Input: part model. Units: mm. Frame: model coordinates. A direction names the side the tool comes from. Give positions to 0.01 mm unless a question says otherwise; leave off trailing zeros. Order: outer loops, then holes, each group sorted by start corner. A loop starts at its lowest first (then second) coordinate and runs counter-clockwise, first axis right, second up. Notation, with made-up numbers: M -31,-5.75 L -7,-5.75 A15 ccw -7,19.25 Z; hole C 39,59 d10. An arc over 180 degrees is marked long. Use a Markdown table: item, result.
from build123d import *

# Parameters (mm, degrees)
F0_W     = 76.2
F0_H     = 76.2
F2_DEPTH = 6.35
F3_DEPTH = 6.35
F4_R     = 2.54
F6_DEPTH = 2.778125
F7_W     = 13.096875
F7_H     = 6.746875
F8_DEPTH = 0.79375


with BuildPart() as f2:
    # F0 (on Top) → F2 (new body)
    with BuildSketch(Plane.XY):
        Rectangle(F0_W, F0_H)
    extrude(amount=-F2_DEPTH)

    # F1 (on Front) → F3 (join, symmetric)
    with BuildSketch(Plane.XZ):
        with BuildLine():
            Line((18.7292598667, 44.45), (25.3953712381, 51.2535714286))
            ThreePointArc((25.3953712381, 51.2535714286), (-28.575, 28.575), (25.3953712381, 5.8964285714))
            Line((25.3953712381, 5.8964285714), (18.7292598667, 12.7))
            ThreePointArc((18.7292598667, 12.7), (-19.05, 28.575), (18.7292598667, 44.45))
        make_face()
    extrude(amount=F3_DEPTH, both=True)

    # F4
    f4_edges = [f2.edges().sort_by_distance(p)[0] for p in [
        (25.395371, 0, 51.253571),
        (18.72926, 0, 44.45),
        (18.72926, 0, 12.7),
        (25.395371, 0, 5.896429),
        (3.175, -6.35, 0),
        (3.175, 6.35, 0),
    ]]
    fillet(f4_edges, radius=F4_R)

    # F5 (on face) → F6 (join)
    with BuildSketch(Plane(origin=(0, 0, -6.35), x_dir=(1, 0, 0), z_dir=(0, 0, -1))):
        Polygon((-38.1, 14.4859375), (-38.1, 23.6140625), (-44.45, 27.2802367094), (-44.45, 10.8197632906), align=None)
        Polygon((-38.1, -23.6140625), (-38.1, -14.4859375), (-44.45, -10.8197632906), (-44.45, -27.2802367094), align=None)
    extrude(amount=-F6_DEPTH)

    # F7 (on face) → F8 (cut)
    with BuildSketch(Plane.XY):
        with Locations((-31.5515625, 9.7234375)):
            Rectangle(F7_W, F7_H)
    extrude(amount=-F8_DEPTH, mode=Mode.SUBTRACT)


solid = f2.part
1) Cut plane B-B on y = 20.5. Return loops of the section in (x, z).
Response values:
| item | result |
|---|---|
| outline | M -44.45,-6.35 L 38.1,-6.35 L 38.1,0 L -38.1,0 L -38.1,-3.57 L -44.45,-3.57 Z |
2) First-contact query: pin 1 Ø16 at (x, z) = (-8, 35.5) entering from -Y; pin 2 Ø5 at (y, z) = (18, 0.5) entering from -X; pin 3 Ø1.9 at (x, y) = (-42.5, 23) entering from +Z; pin 4 Ø7.5 at (x, y) = (-32.5, 9.5) entering from +Z. Flat tips, straight axial feed; report the tip coordinate or a pass-through.
Response values:
| item | result |
|---|---|
| pin 1 | passes through |
| pin 2 | stops at x = -38.1 |
| pin 3 | stops at z = -3.57 |
| pin 4 | stops at z = 0 |
3) Cut plane A-A on x = 18.5. Return loops of the section in (y, z), and give its area (3 significant figures).
Response values:
| item | result |
|---|---|
| outline | M -38.1,-6.35 L 38.1,-6.35 L 38.1,0 L -38.1,0 Z; M -7.07,0.77 L 7.07,0.77 A2.54 cw 6.35,2.54 L 6.35,11.74 L -6.35,11.74 L -6.35,2.54 A2.54 cw Z; M -6.35,45.41 L 6.35,45.41 L 6.35,56.38 L -6.35,56.38 Z |
| area | 763 mm² |
4) Cut plane D-D on x = -8. Return loops of the section in (y, z), and give its area (3 significant figures).
Response values:
| item | result |
|---|---|
| outline | M -38.1,-6.35 L 38.1,-6.35 L 38.1,0 L 8.89,0 A2.54 cw 6.35,2.54 L 6.35,9.36 L -6.35,9.36 L -6.35,2.54 A2.54 cw -8.89,0 L -38.1,0 Z; M -6.35,47.79 L 6.35,47.79 L 6.35,58.29 L -6.35,58.29 Z |
| area | 739 mm² |
5) Material intervals for line 1 (Z direction, x = 17, y = -26.5); line 2 (Z direction, x = 14, y = -0.5); line 3 (Y direction, x = -24, z = 13.5), sorted ascending. Write a range as from..to.
Response values:
| item | result |
|---|---|
| line 1 | z = -6.35..0 |
| line 2 | z = -6.35..9.16, 47.99..58.42 |
| line 3 | y = -6.35..6.35 |
6) Reachability of faces 5 (the face through (18.784, 0.089, 45.415)), 6 (the face through (-32, 10, -0.794)), 7 (the face through (-41.23, -25.42, -4.98)), 8 (the face through (22, -0.09, 9.36)), 9 (the face through (-41.319, -12.627, -4.98)) from +Z, -Z, +X, -X, +Y, -Y: full face, straight path, thin tool, end or side. Return the list, or none.
Response values:
| item | result |
|---|---|
| face 5 | +Y, -Y |
| face 6 | +Z, -X |
| face 7 | +Z, -Z, -Y |
| face 8 | +X, +Y, -Y |
| face 9 | +Z, -Z |
7) Cut plane C-C on z = 47.5. Return loops of the section in (x, y), and give its area (3 significant figures).
Response values:
| item | result |
|---|---|
| outline | M -22.32,-6.35 L -8.48,-6.35 L -8.48,6.35 L -22.32,6.35 Z; M 14.83,-6.35 L 21.72,-6.35 L 21.72,6.35 L 14.83,6.35 Z |
| area | 263 mm² |
8) Mould query, pull axis X, two halves, no side actions, for faces 1 (the face through (21.956, -0.089, 47.743)), 2 (the face through (-41.319, 25.473, -4.98)), 3 (the face through (-14, -6.35, 45)), 4 (the face through (-44.45, -19, -5)). Classes: released by +X, released by -X, zero draft, split by the parting line, or undercut.
Response values:
| item | result |
|---|---|
| face 1 | released by +X |
| face 2 | undercut |
| face 3 | zero draft |
| face 4 | released by -X |
